Input: part model. Units: mm. Frame: model coordinates. Face numbers are marked on the shaded views. Coordinates: 2 decimals unless noted, no trailing zeros. Loops run counter-clockwise (first coordinate to the right, second up) from the corner with the lowest first, then second, coordinate; pieces in that order, holes last. Notation, with made-up numbers: M 19.5,33.25 L 51.5,33.25 A28 ccw 51.5,56.25 Z; hole C 9,47.5 d11. An arc over 180 degrees is marked long. Use a Markdown table: item, result. Add a question column.
1. Section B-B on y = 13. Output: boundary loops of the cut face in (x, z).
2. Section C-C on z = 1. State how many separate pieces and enclosed holes the cut face has, then the cut area to 3 significant figures.
3. Draft query along X for the marked faces 1, 2, 3 and 4. Return one class per face: +X half, -X half, draft (parallel to the pull), parting line (faces both ways), or undercut.
4. Section A-A on x = 0. Output: boundary loops of the cut face in (y, z), then the cut area to 3 significant figures.
5. Section D-D on y = 33. Output: boundary loops of the cut face in (x, z), then the cut area to 3 significant figures.
6. Line query: L1, parallel to Y at x = 0, z = -1.75; L2, parallel to Y at x = -12, z = 0; L3, parallel to Y at x = 7, z = 4.5. Output: solid intervals per line, ascending. Write a range as [from, to].
7. Pin query (flat end, axial travel): pin 1 (2 mm diameter, centred on x = 6.5, y = 47.13, fed in from -Z); pin 2 (1.5 mm diameter, centred on y = 30, z = -3, fed in from -X); pin 3 (1 mm diameter, centred on x = -4.5, z = -1.5, fed in from -Y); pin 4 (4 mm diameter, centred on x = -7, z = 0, fed in from +Y). Return the tip coordinate at first contact, or that it passes through.
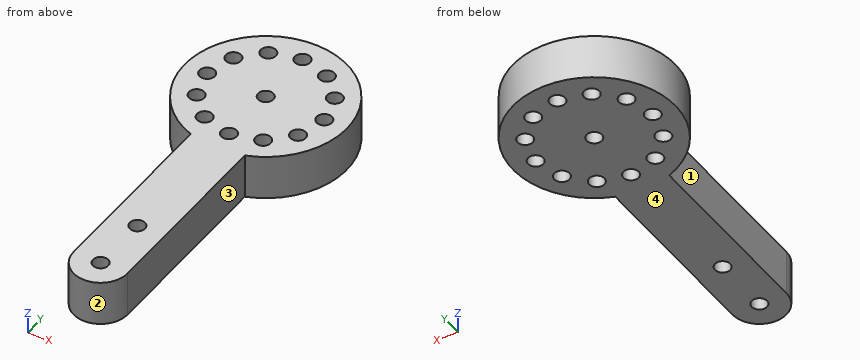
```python
from build123d import *

# Parameters (mm, degrees)
SKETCH1_R           = 1.7
BOSS_EXTRUDE1_DEPTH = 5


with BuildPart() as part:
    # Sketch1 → Boss-Extrude1 (new, symmetric)
    with BuildSketch(Plane.XY):
        with BuildLine():
            Line((-6, 9.245e-06), (-5.999970251, 41.417257276))
            ThreePointArc((-5.999970251, 41.417257276), (-3.1553e-05, 76.387830542), (6.000029749, 41.417278312))
            Line((6.000029749, 41.417278312), (6, -1.1791e-05))
            ThreePointArc((6, -1.1791e-05), (-1.0518e-05, -6), (-6, 9.245e-06))
        make_face()
        Circle(SKETCH1_R, mode=Mode.SUBTRACT)
        with Locations((0, 13)):
            Circle(SKETCH1_R, mode=Mode.SUBTRACT)
        with Locations((0, 58.387830542)):
            Circle(SKETCH1_R, mode=Mode.SUBTRACT)
        with Locations((0, 45.387830542)):
            Circle(SKETCH1_R, mode=Mode.SUBTRACT)
        with Locations((-6.5, 47.129500293)):
            Circle(SKETCH1_R, mode=Mode.SUBTRACT)
        with Locations((-11.258330249, 51.887830542)):
            Circle(SKETCH1_R, mode=Mode.SUBTRACT)
        with Locations((-13, 58.387830542)):
            Circle(SKETCH1_R, mode=Mode.SUBTRACT)
        with Locations((-11.258330249, 64.887830542)):
            Circle(SKETCH1_R, mode=Mode.SUBTRACT)
        with Locations((-6.5, 69.646160791)):
            Circle(SKETCH1_R, mode=Mode.SUBTRACT)
        with Locations((0, 71.387830542)):
            Circle(SKETCH1_R, mode=Mode.SUBTRACT)
        with Locations((6.5, 69.646160791)):
            Circle(SKETCH1_R, mode=Mode.SUBTRACT)
        with Locations((11.258330249, 64.887830542)):
            Circle(SKETCH1_R, mode=Mode.SUBTRACT)
        with Locations((13, 58.387830542)):
            Circle(SKETCH1_R, mode=Mode.SUBTRACT)
        with Locations((11.258330249, 51.887830542)):
            Circle(SKETCH1_R, mode=Mode.SUBTRACT)
        with Locations((6.5, 47.129500293)):
            Circle(SKETCH1_R, mode=Mode.SUBTRACT)
    extrude(amount=BOSS_EXTRUDE1_DEPTH, both=True)


solid = part.part
```
Answers below:
| question | item | result |
|---|---|---|
| 1 | outline | M -6,-5 L -1.7,-5 L -1.7,5 L -6,5 Z; M 1.7,-5 L 6,-5 L 6,5 L 1.7,5 Z |
| 2 | separate pieces | 1 |
| 2 | enclosed holes | 15 |
| 2 | area | 1,430 mm² |
| 3 | face 1 | -X half |
| 3 | face 2 | parting line |
| 3 | face 3 | +X half |
| 3 | face 4 | draft |
| 4 | outline | M -6,-5 L -1.7,-5 L -1.7,5 L -6,5 Z; M 1.7,-5 L 11.3,-5 L 11.3,5 L 1.7,5 Z; M 14.7,-5 L 43.69,-5 L 43.69,5 L 14.7,5 Z; M 47.09,-5 L 56.69,-5 L 56.69,5 L 47.09,5 Z; M 60.09,-5 L 69.69,-5 L 69.69,5 L 60.09,5 Z; M 73.09,-5 L 76.39,-5 L 76.39,5 L 73.09,5 Z |
| 4 | area | 654 mm² |
| 5 | outline | M -6,-5 L 6,-5 L 6,5 L -6,5 Z |
| 5 | area | 120 mm² |
| 6 | L1 | y = [-6, -1.7], [1.7, 11.3], [14.7, 43.69], [47.09, 56.69], [60.09, 69.69], [73.09, 76.39] |
| 6 | L2 | y = [44.97, 50.36], [53.42, 57.01], [59.76, 63.36], [66.42, 71.8] |
| 6 | L3 | y = [41.8, 45.5], [48.75, 68.02], [71.27, 74.97] |
| 7 | pin 1 | passes through |
| 7 | pin 2 | stops at x = -6 |
| 7 | pin 3 | stops at y = -4.47 |
| 7 | pin 4 | stops at y = 75.68 |
